```python
from build123d import *

# Parameters (mm, degrees)
F0_W     = 25
F0_H     = 25
F0_W_2   = 21
F0_H_2   = 21
F1_DEPTH = 380
F2_R     = 2.5
F3_DEPTH = 25
F4_R     = 2.5
F5_DEPTH = 25


with BuildPart() as f1:
    # F0 (on Top) → F1 (new body)
    with BuildSketch(Plane.XY):
        Rectangle(F0_W, F0_H)
        Rectangle(F0_W_2, F0_H_2, mode=Mode.SUBTRACT)
    extrude(amount=F1_DEPTH)

    # F2 (on face) → F3 (cut)
    with BuildSketch(Plane.XZ.offset(12.5)):
        with Locations((0, 372)):
            Circle(F2_R)
        with Locations((0, 7.5)):
            Circle(F2_R)
    extrude(amount=-F3_DEPTH, mode=Mode.SUBTRACT)

    # F4 (on face) → F5 (cut)
    with BuildSketch(Plane.YZ.offset(12.5)):
        with Locations((0, 372)):
            Circle(F4_R)
        with Locations((0, 7.5)):
            Circle(F4_R)
    extrude(amount=-F5_DEPTH, mode=Mode.SUBTRACT)


solid = f1.part
```
Geometry check sheet. Reference: the model listing, model coordinates, mm. A direction names the side the tool comes from. Round coordinates to 2 decimals unless told otherwise and drop trailing zeros. Write each loop counter-clockwise with the first axis right and the second up, starting at its lowest first coordinate (ties: lowest second). Pieces come first, ordered by that corner, then holes. Notation, with made-up numbers: (57.25, 83) -> (88.25, 83) arc R23 cw to (88.25, 94) -> close; hole circle Ø9 at (4, 75.5). An arc over 180 degrees is marked (long way). Put each result on its own line as item: value.
1) Cross-section at B-B, the plane z = 176.5. Enter the section's corners in (x, y), plus the area to 3 significant figures.
Recorded:
outline: (-12.5, -12.5) -> (12.5, -12.5) -> (12.5, 12.5) -> (-12.5, 12.5) -> close; hole (-10.5, -10.5) -> (10.5, -10.5) -> (10.5, 10.5) -> (-10.5, 10.5) -> close
area: 184 mm2
2) Access from +Z, -Z, +X, -X, +Y, -Y to the whole of each face (thin tool, end or side, straight path). Record for faces 5 (the face through (-11, 0, 380)), 6 (the face through (-10.5, 0, 187)).
Recorded:
face 5: +Z, +X, -X, +Y, -Y
face 6: +Z, -Z
3) Cross-section at A-A, the plane x = -7. Enter the section's corners in (y, z), plus the area to 3 significant figures.
Recorded:
outline: (-12.5, 0) -> (-10.5, 0) -> (-10.5, 380) -> (-12.5, 380) -> close; (10.5, 0) -> (12.5, 0) -> (12.5, 380) -> (10.5, 380) -> close
area: 1,520 mm2
4) Thickness scan on probe 1 along Z at (x, y) = (0, 11.8); probe 2 along Y at (x, z) = (8.25, 67). Record the ranges inside material, lowest first. Write a range as from..to.
Recorded:
probe 1: z = 0..5, 10..369.5, 374.5..380
probe 2: y = -12.5..-10.5, 10.5..12.5
5) Release check for a two-part mould opening along X. For faces 1 (the face through (-12.5, 0, 187)), 2 (the face through (0, -10.5, 187)), 3 (the face through (0, 12.5, 187)), 4 (the face through (12.5, 0, 187)) record: pulls with the +X half, pulls with the -X half, needs draft (parallel to the pull), parting line crosses it, or undercut.
Recorded:
face 1: pulls with the -X half
face 2: undercut
face 3: needs draft
face 4: pulls with the +X half
